from build123d import *

# Parameters (mm, degrees)
SKETCH1_R               = 3.475
SKETCH1_R_2             = 2.3828
BOSS_EXTRUDE1_DEPTH     = 6.35
CHAMFER1_SIZE           = 3
CHAMFER2_SIZE           = 8
CUT_EXTRUDE1_DEPTH      = 2.286
CUT_EXTRUDE2_DEPTH      = 36.817152344
CUT_EXTRUDE2_DEPTH_BACK = 36.817152344
SKETCH4_W               = 40.986
SKETCH4_H               = 20.158
SKETCH6_W               = 57.000074061
SKETCH6_H               = 19.05
CUT_EXTRUDE3_DEPTH      = 37.147957148
SKETCH9_W               = 40.986
SKETCH9_H               = 4.397387502
BOSS_EXTRUDE2_DEPTH     = 25.4
CHAMFER3_SIZE           = 2.54
SKETCH10_W              = 3.175
SKETCH10_H              = 31.75
BOSS_EXTRUDE3_DEPTH     = 6.35
SKETCH11_R              = 5.55625
CUT_EXTRUDE4_DEPTH      = 3
SKETCH14_R              = 2.58125
CUT_EXTRUDE10_DEPTH     = 6.35
CHAMFER4_SIZE           = 0.4


with BuildPart() as part:
    # Sketch1 → Boss-Extrude1 (new body)
    with BuildSketch(Plane.XY):
        Polygon((17.4625, -21.209), (-17.4625, -21.209), (-17.4625, 1.651), (-28.575, 1.651), (-28.575, 21.209), (28.575, 21.209), (28.575, 1.651), (17.4625, 1.651), align=None)
        with Locations((-9.525, -10.541)):
            Circle(SKETCH1_R, mode=Mode.SUBTRACT)
        with Locations((9.525, -10.541)):
            Circle(SKETCH1_R, mode=Mode.SUBTRACT)
        with Locations((-24.13, 6.35)):
            Circle(SKETCH1_R_2, mode=Mode.SUBTRACT)
        with Locations((-24.13, 16.51)):
            Circle(SKETCH1_R_2, mode=Mode.SUBTRACT)
        with Locations((24.13, 16.51)):
            Circle(SKETCH1_R_2, mode=Mode.SUBTRACT)
        with Locations((24.13, 6.35)):
            Circle(SKETCH1_R_2, mode=Mode.SUBTRACT)
    extrude(amount=BOSS_EXTRUDE1_DEPTH)

    # Chamfer1
    chamfer1_edges = [part.edges().sort_by_distance(p)[0] for p in [
        (-28.575, 1.651, 3.175),
        (-28.575, 21.209, 3.175),
        (28.575, 21.209, 3.175),
        (28.575, 1.651, 3.175),
        (17.4625, -21.209, 3.175),
        (-17.4625, -21.209, 3.175),
    ]]
    chamfer(chamfer1_edges, length=CHAMFER1_SIZE)

    # Chamfer2
    chamfer2_edges = [part.edges().sort_by_distance(p)[0] for p in [
        (17.4625, 1.651, 3.175),
        (-17.4625, 1.651, 3.175),
    ]]
    chamfer(chamfer2_edges, length=CHAMFER2_SIZE)

    # Sketch3 → Cut-Extrude1 (cut)
    with BuildSketch(Plane.XY.offset(6.35)):
        Polygon((-25.4625, 1.651), (25.4625, 1.651), (25.575, 1.651), (28.575, 4.651), (28.575, 18.209), (25.575, 21.209), (-25.575, 21.209), (-28.575, 18.209), (-28.575, 4.651), (-25.575, 1.651), align=None)
    extrude(amount=-CUT_EXTRUDE1_DEPTH, mode=Mode.SUBTRACT)

    # Sketch4 → Cut-Extrude2 (cut, two sides: drawn at the far end of the back side and taken through both)
    with BuildSketch(Plane.XY.offset(4.064).offset(-CUT_EXTRUDE2_DEPTH_BACK)):
        with Locations((0, 11.43)):
            Rectangle(SKETCH4_W, SKETCH4_H)
    extrude(amount=CUT_EXTRUDE2_DEPTH + CUT_EXTRUDE2_DEPTH_BACK, mode=Mode.SUBTRACT)

    # Sketch6 → Cut-Extrude3 (cut, through all)
    with BuildSketch(Plane.XY.offset(6.35)):
        with Locations((-1.923625946, -12.571387502)):
            Rectangle(SKETCH6_W, SKETCH6_H)
    extrude(amount=-CUT_EXTRUDE3_DEPTH, mode=Mode.SUBTRACT)

    # Sketch9 → Boss-Extrude2 (add)
    with BuildSketch(Plane(origin=(0, 0, 0), x_dir=(-1, 0, 0), z_dir=(0, 0, -1))):
        with Locations((0, -0.847693751)):
            Rectangle(SKETCH9_W, SKETCH9_H)
    extrude(amount=BOSS_EXTRUDE2_DEPTH)

    # Chamfer3
    chamfer3_edges = [part.edges().sort_by_distance(p)[0] for p in [
        (-20.493, -0.847693751, 0),
        (20.493, -0.847693751, 0),
    ]]
    chamfer(chamfer3_edges, length=CHAMFER3_SIZE)

    # Sketch10 → Boss-Extrude3 (add)
    with BuildSketch(Plane(origin=(0, -3.046387502, 0), x_dir=(-1, 0, 0), z_dir=(0, -1, 0))):
        with Locations((18.9055, 9.525)):
            Rectangle(SKETCH10_W, SKETCH10_H)
        with Locations((-9.9695, 9.525)):
            Rectangle(SKETCH10_W, SKETCH10_H)
    extrude(amount=BOSS_EXTRUDE3_DEPTH)

    # Sketch11 → Cut-Extrude4 (cut)
    with BuildSketch(Plane(origin=(0, 1.351, 0), x_dir=(1, 0, 0), z_dir=(0, 1, 0))):
        with Locations(Location((0, 0, 0), (0, 0, 180))):
            Circle(SKETCH11_R)
    extrude(amount=-CUT_EXTRUDE4_DEPTH, mode=Mode.SUBTRACT)

    # Sketch14 → Cut-Extrude10 (cut)
    with BuildSketch(Plane(origin=(0, -1.649, 0), x_dir=(1, 0, 0), z_dir=(0, 1, 0))):
        with Locations(Location((0, 0, 0), (0, 0, 180))):
            Circle(SKETCH14_R)
    extrude(amount=-CUT_EXTRUDE10_DEPTH, mode=Mode.SUBTRACT)

    # Chamfer4
    chamfer4_edges = [part.edges().sort_by_distance(p)[0] for p in [
        (5.55625, 1.351, 0),
    ]]
    chamfer(chamfer4_edges, length=CHAMFER4_SIZE)


solid = part.part
Geometry: final body of the model. Coordinates: model frame, mm. A direction names the side the tool comes from. Coordinates: 2 decimals unless noted, no trailing zeros. Order: outer loops, then holes, each group sorted by start corner. A loop starts at its lowest first (then second) coordinate and runs counter-clockwise, first axis right, second up.
(1) Access query for faces 5 (the face through (4.095, -0.331, 3.755)), 6 (the face through (16, -3.046, -9)), 7 (the face through (24, 12, 4.064)), 8 (the face through (-27.054, 19.73, 2.004)), 9 (the face through (20.493, -1, -14)). Directions: +Z, -Z, +X, -X, +Y, -Y. A direction counts if a zero-diameter tool reaches every point of the face in a straight line with its end or side. Return the directions, or none.
(2) Section query C-C (x = -13). Return the cut outline in (y, z), plus the area to 3 significant figures.
(3) Section query B-B (z = -14). Return the cut outline in (x, y).
(4) Draft query along X for faces 1 (the face through (11.557, -6, -9)), 2 (the face through (-21.929, 5.437, 2.004)), 3 (the face through (-5, 1.351, -9)), 4 (the face through (-25, 12, 4.064)). Return one class per face: pulls with the +X half, pulls with the -X half, needs draft (parallel to the pull), parting line crosses it, or undercut.
(5) Section query A-A (y = 16.51). Return the cut outline in (x, z) (3 decimals), plus the area to 3 significant figures.
(6) First-contact query: pin 1 (8 mm diameter, centred on y = -3.5, z = -5, fed in from -X); pin 2 (1 mm diameter, centred on x = 18.5, z = -4, fed in from -Y); pin 3 (2.5 mm diameter, centred on x = -23, y = 13, fed in from +Z); pin 4 (3 mm diameter, centred on x = -24.13, y = 16.51, fed in from +Z). Flat tips, straight axial feed; report the tip coordinate or a pass-through.
(7) Section query D-D (y = 7). Return the cut outline in (x, z) (3 decimals).
(8) Material intervals for probe 1 along X at (y, z) = (6.35, 0.95) (3 decimals); probe 2 along Y at (x, z) = (-24.13, 1.15); probe 3 along X at (y, z) = (17, 1.5) (3 decimals), sorted ascending.
Solution:
1. face 5: +Y
1. face 6: +Z, -Z, +X, -Y
1. face 7: +Z, +X, -X, +Y
1. face 8: +Z, -Z, -X, +Y
1. face 9: -Z, +X, +Y, -Y
2. outline: (-3.05, -25.4) - (1.35, -25.4) - (1.35, 6.35) - (-3.05, 6.35) - close
2. area: 140 mm2
3. outline: (-20.49, -9.4) - (-17.32, -9.4) - (-17.32, -3.05) - (8.38, -3.05) - (8.38, -9.4) - (11.56, -9.4) - (11.56, -3.05) - (20.49, -3.05) - (20.49, 1.35) - (-20.49, 1.35) - close
4. face 1: pulls with the +X half
4. face 2: undercut
4. face 3: undercut
4. face 4: needs draft
5. outline: (-28.575, 0) - (-26.513, 0) - (-26.513, 4.064) - (-28.575, 4.064) - close; (-21.747, 0) - (-20.493, 0) - (-20.493, 4.064) - (-21.747, 4.064) - close; (20.493, 0) - (21.747, 0) - (21.747, 4.064) - (20.493, 4.064) - close; (26.513, 0) - (28.575, 0) - (28.575, 4.064) - (26.513, 4.064) - close
5. area: 27.0 mm2
6. pin 1: stops at x = -21.76
6. pin 2: stops at y = -3.05
6. pin 3: stops at z = 4.06
6. pin 4: passes through
7. outline: (-28.575, 0) - (-26.422, 0) - (-26.422, 4.064) - (-28.575, 4.064) - close; (-21.838, 0) - (-20.493, 0) - (-20.493, 4.064) - (-21.838, 4.064) - close; (20.493, 0) - (21.838, 0) - (21.838, 4.064) - (20.493, 4.064) - close; (26.422, 0) - (28.575, 0) - (28.575, 4.064) - (26.422, 4.064) - close
8. probe 1: x = -28.575 to -26.513, -21.747 to -20.493, 20.493 to 21.747, 26.513 to 28.575
8. probe 2: y = 0.32 to 3.97, 8.73 to 14.13, 18.89 to 21.21
8. probe 3: x = -28.575 to -26.462, -21.798 to -20.493, 20.493 to 21.798, 26.462 to 28.575
